```python
from build123d import *

# Parameters (mm, degrees)
F1_DEPTH = 31
F2_R     = 1.808584
F3_DEPTH = 25
F5_DEPTH = 25


with BuildPart() as f1:
    # F0 (on Top) → F1 (new body)
    with BuildSketch(Plane.XY):
        with BuildLine():
            Line((-4.311411, 30.573439), (-4.311411, 43.788447))
            Line((-4.311411, 43.788447), (-9.311411, 43.788447))
            Line((-9.311411, 43.788447), (-9.311411, 33.390859))
            ThreePointArc((-9.311411, 33.390859), (-15.293246, 18.476209), (-4.837364, 6.273601))
            Line((-4.837364, 6.273601), (-8.5, 6.273601))
            Line((-8.5, 6.273601), (-8.5, -45.726399))
            Line((-8.5, -45.726399), (-7, -45.726399))
            Line((-7, -45.726399), (7, -45.726399))
            Line((7, -45.726399), (8.5, -45.726399))
            Line((8.5, -45.726399), (8.5, 6.273601))
            Line((8.5, 6.273601), (4.837364, 6.273601))
            ThreePointArc((4.837364, 6.273601), (15.293246, 18.476209), (9.311411, 33.390859))
            Line((9.311411, 33.390859), (9.311411, 43.788447))
            Line((9.311411, 43.788447), (4.311411, 43.788447))
            Line((4.311411, 43.788447), (4.311411, 30.573439))
            ThreePointArc((4.311411, 30.573439), (10.367578, 19.337097), (1.102061, 10.557421))
            ThreePointArc((1.102061, 10.557421), (0.551793, 10.513934), (0, 10.499425))
            ThreePointArc((0, 10.499425), (-0.551793, 10.513934), (-1.102061, 10.557421))
            ThreePointArc((-1.102061, 10.557421), (-10.367578, 19.337097), (-4.311411, 30.573439))
        make_face()
    extrude(amount=F1_DEPTH)

    # F2 (on face) → F3 (cut)
    with BuildSketch(Plane(origin=(-9.311411, 0, 0), x_dir=(0, -1, 0), z_dir=(-1, 0, 0))):
        with Locations((-39.933514, 15.5)):
            Circle(F2_R)
    extrude(amount=-F3_DEPTH, mode=Mode.SUBTRACT)

    # F4 (on face) → F5 (cut)
    with BuildSketch(Plane(origin=(-8.5, 0, 0), x_dir=(0, -1, 0), z_dir=(-1, 0, 0))):
        Polygon((40.726399, 5), (40.726399, 13), (45.726399, 13), (45.726399, 18), (40.726399, 18), (40.726399, 26), (-1.273601, 26), (-1.273601, 5), align=None)
    extrude(amount=-F5_DEPTH, mode=Mode.SUBTRACT)


solid = f1.part
```
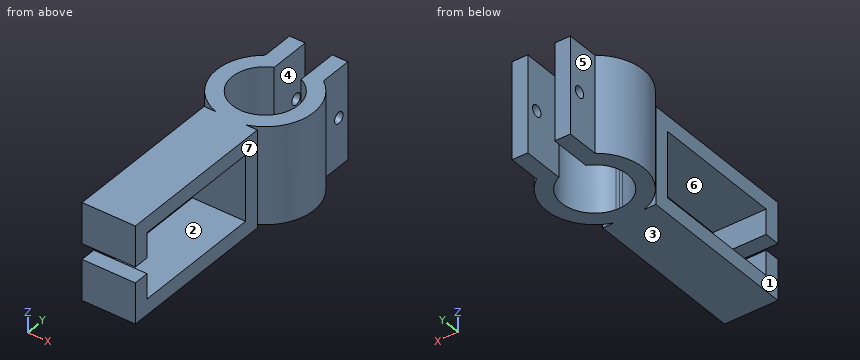
For this review, take the finished solid that the model builds, in its own axes (mm). Face numbers are marked on the shaded views. A direction names the side the tool comes from. Coordinates: 2 decimals unless noted, no trailing zeros. Write each loop counter-clockwise with the first axis right and the second up, starting at its lowest first coordinate (ties: lowest second). Pieces come first, ordered by that corner, then holes.
(1) The part is to be moulded in two halves that separate along Z. For the marked faces 1, 2 and 3, say which applies: +Z half, -Z half, draft (parallel to the pull), parting line (faces both ways), or undercut.
(2) Add section A-A on z = 22.5. Give the boundary of the cut face in (x, y).
(3) For pin 1 Ø12 at (y, z) = (3.5, 18) entering from -X; pin 2 Ø11.5 at (y, z) = (36, 16.5) entering from +X; pin 3 Ø2.5 at (x, z) = (1.5, 9.5) entering from +Y, all flat-tipped, find the tip position at first contact; note any pin that passes through.
(4) Tool access review of the marked faces 4, 5, 6 and 7: name each direction out of +Z, -Z, +X, -X, +Y, -Y from which nothing blocks a thin tool from reaching the whole face with its end or side.
(5) Add section D-D on z = 15.5. Give the boundary of the cut face in (x, y).
(6) Add section B-B on y = -26. Give the boundary of the cut face in (x, z), then the cut area to 3 significant figures.
(7) Wall thickness on probe 1 along Z at (x, y) = (7, -38); probe 2 along X at (y, z) = (20.5, 28); probe 3 along X at (y, z) = (-14.5, 4.5): over which ranges is each line inside the solid? List them lowest first.
(8) Add section C-C on x = -6.5. Give the boundary of the cut face in (y, z).
Answer sheet:
1. face 1: draft
1. face 2: undercut
1. face 3: -Z half
2. outline: (-9.31, 33.39) arc R15.5 ccw to (-4.84, 6.27) - (-8.5, 6.27) - (-8.5, 1.27) - (8.5, 1.27) - (8.5, 6.27) - (4.84, 6.27) arc R15.5 ccw to (9.31, 33.39) - (9.31, 43.79) - (4.31, 43.79) - (4.31, 30.57) arc R10.5 cw to (1.1, 10.56) arc R10.5 cw to (0, 10.5) arc R10.5 cw to (-1.1, 10.56) arc R10.5 cw to (-4.31, 30.57) - (-4.31, 43.79) - (-9.31, 43.79) - close; (-8.5, -45.73) - (8.5, -45.73) - (8.5, -40.73) - (-8.5, -40.73) - close
3. pin 1: stops at x = -10.39
3. pin 2: stops at x = 12.44
3. pin 3: stops at y = 10.87
4. face 4: +Z, -Z, +Y
4. face 5: +Z, -Z, -X, +Y
4. face 6: +X, -X
4. face 7: +Z, -Z, +X, -Y
5. outline: (-9.31, 33.39) arc R15.5 ccw to (-4.84, 6.27) - (-8.5, 6.27) - (-8.5, 1.27) - (8.5, 1.27) - (8.5, 6.27) - (4.84, 6.27) arc R15.5 ccw to (9.31, 33.39) - (9.31, 38.12) - (4.31, 38.12) - (4.31, 30.57) arc R10.5 cw to (1.1, 10.56) arc R10.5 cw to (0, 10.5) arc R10.5 cw to (-1.1, 10.56) arc R10.5 cw to (-4.31, 30.57) - (-4.31, 38.12) - (-9.31, 38.12) - close; (-9.31, 41.74) - (-4.31, 41.74) - (-4.31, 43.79) - (-9.31, 43.79) - close; (4.31, 41.74) - (9.31, 41.74) - (9.31, 43.79) - (4.31, 43.79) - close
6. outline: (-8.5, 0) - (8.5, 0) - (8.5, 5) - (-8.5, 5) - close; (-8.5, 26) - (8.5, 26) - (8.5, 31) - (-8.5, 31) - close
6. area: 170 mm2
7. probe 1: z = 0 to 5, 26 to 31
7. probe 2: x = -15.49 to -10.49, 10.49 to 15.49
7. probe 3: x = -8.5 to 8.5
8. outline: (-45.73, 0) - (6.27, 0) - (6.27, 31) - (-45.73, 31) - (-45.73, 18) - (-40.73, 18) - (-40.73, 26) - (1.27, 26) - (1.27, 5) - (-40.73, 5) - (-40.73, 13) - (-45.73, 13) - close; (6.93, 0) - (12.75, 0) - (12.75, 31) - (6.93, 31) - close; (29.25, 0) - (43.79, 0) - (43.79, 31) - (29.25, 31) - close; hole circle Ø3.62 at (39.93, 15.5)
